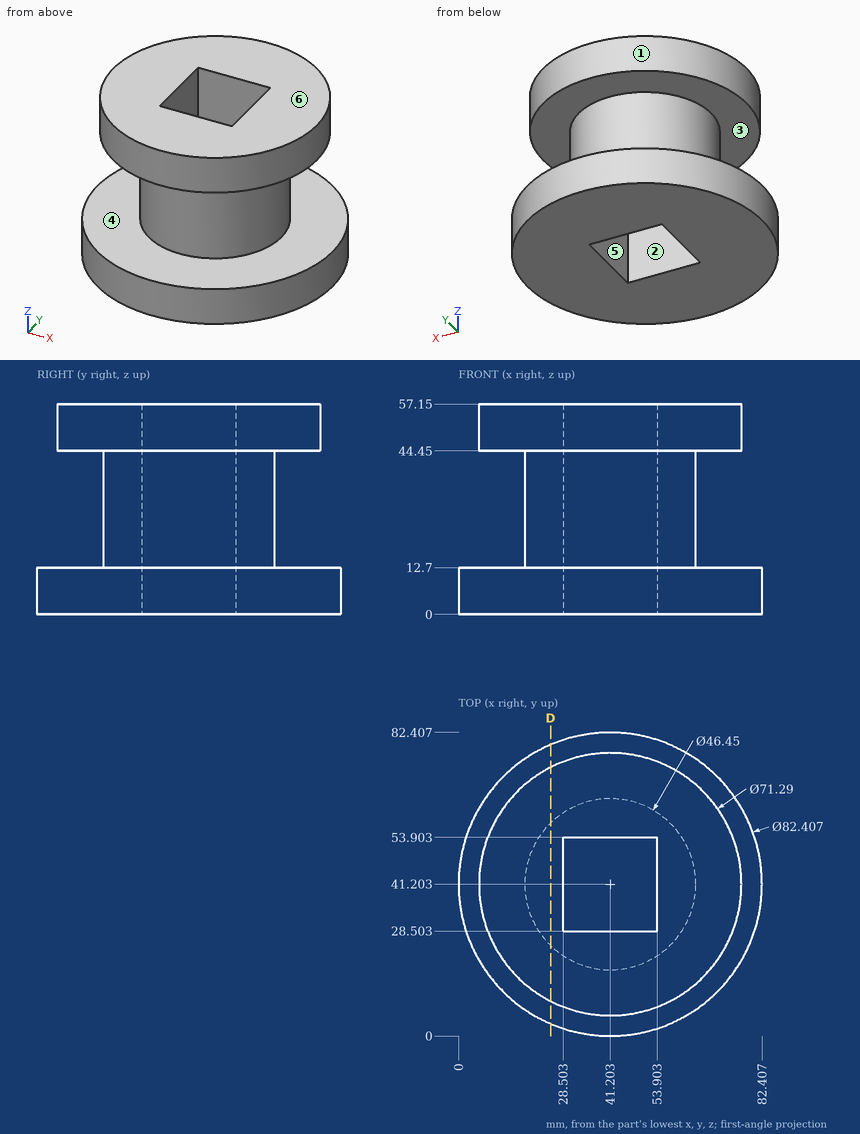
Verification items for this drawing (mm, ordinates from the low corner). A direction names the side the tool comes from. Give positions to 0.01 mm unless a question says otherwise; leave off trailing zeros. Loops run counter-clockwise (first coordinate to the right, second up) from the corner with the lowest first, then second, coordinate; pieces in that order, holes last. Notation, with made-up numbers: M -15.75,72 L 16.25,72 A18 cw 16.25,97 Z; hole C 76.5,36 d1. An arc over 180 degrees is marked long. Write item = value, one per line. Start each with the question number.
1. Thickness scan on probe 1 along Z at (x, y) = (21, 53); probe 2 along Z at (x, y) = (75, 60); probe 3 along Y at (x, z) = (38.5, 33). Record the ranges inside material, lowest first.
2. Go/stop test with flat-tipped pins: P1, Ø10, axis at y = 18, z = 10.5, coming from the -X side; P2, Ø20.5, axis at y = 37, z = 30, coming from the +X side; P3, Ø10, axis at y = 34, z = 10, coming from the +X side; P4, Ø1.5, axis at x = 70.5, z = 14, coming from the -Y side. Record where each tip stops, or that it passes through.
3. Tool access check on the marked faces 4, 5 and 6. Record the directions out of +Z, -Z, +X, -X, +Y, -Y that give a thin tool (end or side, any length) a straight path to the whole face; none if there is none.
4. Draft check along Y on the marked faces 1, 2 and 3. Enter one of: +Y half, -Y half, draft (parallel to the pull), parting line (faces both ways), or undercut.
5. Section check D-D, the plane x = 25. Enter the section's corners in (y, z), plus the area to 3 significant figures.
Values follow:
q1.probe_1 = 0 to 12.7, 44.45 to 57.15
q1.probe_2 = 0 to 12.7
q1.probe_3 = 18.14 to 28.5, 53.9 to 64.27
q2.P1 = 4.24
q2.P2 = 64.43
q2.P3 = 82.35
q2.P4 = through
q3.face_4 = none
q3.face_5 = +Z, -Z
q3.face_6 = +Z, +X, -X, +Y, -Y
q4.face_1 = parting line
q4.face_2 = undercut
q4.face_3 = draft
q5.outline = M 3.32,0 L 79.09,0 L 79.09,12.7 L 57.84,12.7 L 57.84,44.45 L 72.95,44.45 L 72.95,57.15 L 9.45,57.15 L 9.45,44.45 L 24.56,44.45 L 24.56,12.7 L 3.32,12.7 Z
q5.area = 2,830 mm^2
